Design review of the part built by this model. Coordinates are the model's own, in mm. A direction names the side the tool comes from. Give positions to 0.01 mm unless a question says otherwise; leave off trailing zeros. Order: outer loops, then holes, each group sorted by start corner. A loop starts at its lowest first (then second) coordinate and runs counter-clockwise, first axis right, second up. Notation, with made-up numbers: (-1.75, 75.25) -> (7.25, 75.25) arc R31 ccw to (7.25, 99.25) -> close; hole circle Ø1 at (51, 36.5). An arc over 180 degrees is marked (long way). One line per item, written item: value. Start each with the question number.
1) For pin 1 (7.5 mm diameter, centred on y = 0, z = 133.35, fed in from -X), flat-tipped, find the tip position at first contact; note if it passes through.
2) Consider section B-B (x = 2.75). State the section outline as (y, z) points, plus the area to 3 significant figures.
3) Tool access review of faces 1 (the face through (-11.049, 0, -3)), 2 (the face through (-12.7, 0, -3)): name each direction out of +Z, -Z, +X, -X, +Y, -Y from which nothing blocks a thin tool from reaching the whole face with its end or side.
4) Consider section A-A (y = 19.5). State the section outline as (x, z) points, plus the area to 3 significant figures.
5) The part is to be moulded in two halves that separate along Z. For faces 3 (the face through (-11.3, 2, 190.5)), 4 (the face through (11.863, -1.907, 127.293)), 5 (the face through (12.7, 0, -3)), say which applies: released by +Z, released by -Z, zero draft, split by the parting line, or undercut.
6) Consider section D-D (z = 66). State the section outline as (x, y) points, plus the area to 3 significant figures.
7) Wall thickness on line 1 along Y through (x, z) = (11.8, -133.35); line 2 along X through (y, z) = (-4.5, 122); line 3 along Y through (x, z) = (0.25, -49.5): over which ranges is each line inside the solid? List them lowest first. Write a range as from..to.
8) Consider section C-C (z = 133.35). State the section outline as (x, y) points.
Autodesk Inventor part; units mm, degrees
ref_plane "YZ Plane" through (0, 0, 0) normal (1, 0, 0) x (0, 1, 0)
ref_plane "XY Plane" through (0, 0, 0) normal (0, 0, 1) x (1, 0, 0)
sketch "Sketch1" plane through (0, 0, 0) normal (0, 0, 1) x (1, 0, 0)
  line L0 (-12.7, -25.4) -> (12.7, -25.4)
  line L1 (12.7, -25.4) -> (12.7, 25.4)
  line L2 (12.7, 25.4) -> (-12.7, 25.4)
  line L3 (-12.7, 25.4) -> (-12.7, -25.4)
  line L4 (-12.7, -25.4) -> (12.7, 25.4) construction
  line L5 (12.7, -25.4) -> (-12.7, 25.4) construction
  line L6 (-11.049, -23.749) -> (11.049, -23.749)
  line L7 (11.049, -23.749) -> (11.049, 23.749)
  line L8 (11.049, 23.749) -> (-11.049, 23.749)
  line L9 (-11.049, 23.749) -> (-11.049, -23.749)
  line L10 (-11.049, -23.749) -> (11.049, 23.749) construction
  line L11 (11.049, -23.749) -> (-11.049, 23.749) construction
  point P0 (0, 0)
  dimension "d0" = 25.4
  dimension "d1" = 50.8
  dimension "d4" = 22.098
  dimension "d5" = 47.498
extrude "Extrusion2" add sketch "Sketch1" along normal mid plane 381
sketch "Sketch3" plane through (12.7, -25.4, 190.5) normal (1, 0, 0) x (0, 0, -1)
  line L0 (381, 50.8) -> (0, 50.8)
  line L1 (0, 0) -> (0, 50.8)
  line L2 (381, 0) -> (0, 0)
  line L3 (381, 50.8) -> (381, 0)
  circle A0 centre (57.15, 25.4) radius 6.35
  point P0 (190.5, 25.4)
  dimension "d22" = 12.7
  dimension "d23" = 57.15
  dimension "d24" = 25.4
hole "Hole2" at (12.7, 0, 133.35) direction (-1, 0, 0) diameter 12.7 end through all
sketch "Sketch4" plane through (12.7, -25.4, 190.5) normal (1, 0, 0) x (0, 0, -1)
  circle A0 centre (57.15, 25.4) radius 6.35
  line L0 (381, 50.8) -> (0, 50.8)
  line L1 (0, 0) -> (0, 50.8)
  line L2 (381, 0) -> (0, 0)
  line L3 (381, 50.8) -> (381, 0)
  point P0 (190.5, 25.4)
  point P1 (323.85, 25.4)
  dimension "d32" = 57.15
  dimension "d33" = 25.4
hole "Hole3" at (12.7, 0, -133.35) direction (-1, 0, 0) diameter 12.7 end through all
sketch "Sketch5" plane through (12.7, -25.4, 190.5) normal (1, 0, 0) x (0, 0, -1)
  circle A0 centre (323.85, 25.4) radius 6.35
  circle A1 centre (57.15, 25.4) radius 6.35
  line L0 (381, 50.8) -> (0, 50.8)
  line L1 (0, 0) -> (0, 50.8)
  line L2 (381, 0) -> (0, 0)
  line L3 (381, 50.8) -> (381, 0)
  point P0 (190.5, 25.4)
  point P1 (355.6, 25.4)
  point P2 (292.1, 25.4)
  dimension "d41" = 63.5
  dimension "d42" = 31.75
hole "Hole4" at (12.7, 0, -101.6) at (12.7, 0, -165.1) direction (-1, 0, 0) diameter 5.08 end through all
sketch "Sketch6" plane through (12.7, -25.4, 190.5) normal (1, 0, 0) x (0, 0, -1)
  circle A0 centre (292.1, 25.4) radius 2.54
  circle A1 centre (355.6, 25.4) radius 2.54
  circle A2 centre (323.85, 25.4) radius 6.35
  circle A3 centre (57.15, 25.4) radius 6.35
  line L0 (381, 50.8) -> (0, 50.8)
  line L1 (0, 0) -> (0, 50.8)
  line L2 (381, 0) -> (0, 0)
  line L3 (381, 50.8) -> (381, 0)
  circle A4 centre (38.1, 25.4) radius 2.54
  line L4 (57.15, 31.75) -> (57.15, 19.05) construction
  circle A5 centre (76.2, 25.4) radius 2.54
  point P0 (190.5, 25.4)
  dimension "d53" = 5.08
  dimension "d54" = 19.05
hole "Hole5" at (12.7, 0, 152.4) at (12.7, 0, 114.3) direction (-1, 0, 0) diameter 5.08 end through all
properties part number "Steel 4130 1x2in. Tubing, t=.065in.,L=15in." material "Steel"
Checked values:
1. pin 1: passes through
2. outline: (-25.4, -190.5) -> (-23.75, -190.5) -> (-23.75, 190.5) -> (-25.4, 190.5) -> close; (23.75, -190.5) -> (25.4, -190.5) -> (25.4, 190.5) -> (23.75, 190.5) -> close
2. area: 1,260 mm^2
3. face 1: +Z, -Z
3. face 2: +Z, -Z, -X, +Y, -Y
4. outline: (-12.7, -190.5) -> (-11.05, -190.5) -> (-11.05, 190.5) -> (-12.7, 190.5) -> close; (11.05, -190.5) -> (12.7, -190.5) -> (12.7, 190.5) -> (11.05, 190.5) -> close
4. area: 1,260 mm^2
5. face 3: released by +Z
5. face 4: undercut
5. face 5: zero draft
6. outline: (-12.7, -25.4) -> (12.7, -25.4) -> (12.7, 25.4) -> (-12.7, 25.4) -> close; hole (-11.05, -23.75) -> (11.05, -23.75) -> (11.05, 23.75) -> (-11.05, 23.75) -> close
6. area: 241 mm^2
7. line 1: y = -25.4..-6.35, 6.35..25.4
7. line 2: x = -12.7..-11.05, 11.05..12.7
7. line 3: y = -25.4..-23.75, 23.75..25.4
8. outline: (-12.7, -25.4) -> (12.7, -25.4) -> (12.7, -6.35) -> (11.05, -6.35) -> (11.05, -23.75) -> (-11.05, -23.75) -> (-11.05, -6.35) -> (-12.7, -6.35) -> close; (-12.7, 6.35) -> (-11.05, 6.35) -> (-11.05, 23.75) -> (11.05, 23.75) -> (11.05, 6.35) -> (12.7, 6.35) -> (12.7, 25.4) -> (-12.7, 25.4) -> close
